Part model, mm, in its own coordinate system. A direction names the side the tool comes from. Give positions to 0.01 mm unless a question says otherwise; leave off trailing zeros. Order: outer loops, then holes, each group sorted by start corner. A loop starts at its lowest first (then second) coordinate and runs counter-clockwise, first axis right, second up. Notation, with made-up numbers: M -24.75,79 L -18.75,79 A12 ccw -18.75,91 Z; hole C 9,75 d7. An arc over 180 degrees is marked long. Return JSON: item names as keys, results as strings.
Autodesk Inventor part; units mm, degrees
ref_plane "YZ Plane" through (0, 0, 0) normal (1, 0, 0) x (0, 1, 0)
ref_plane "XZ Plane" through (0, 0, 0) normal (0, 1, 0) x (-1, 0, 0)
ref_plane "XY Plane" through (0, 0, 0) normal (0, 0, 1) x (1, 0, 0)
sketch "Boceto1" plane through (0, 0, 0) normal (1, 0, 0) x (0, 1, 0)
  line L0 (-6.321, 6.321) -> (6.321, 6.321) construction
  line L1 (6.321, 6.321) -> (6.321, -6.321) construction
  line L2 (6.321, -6.321) -> (-6.321, -6.321) construction
  line L3 (-6.321, -6.321) -> (-6.321, 6.321) construction
  line L4 (-6.321, 6.321) -> (6.321, -6.321) construction
  line L5 (6.321, 6.321) -> (-6.321, -6.321) construction
  circle A0 centre (6.321, -6.321) radius 0.875
  line L6 (0, 0) -> (7.9878, 0) construction
  circle A1 centre (6.321, 6.321) radius 0.875
  line L7 (0, 0) -> (0, -13.4562) construction
  circle A2 centre (-6.321, -6.321) radius 0.875
  circle A3 centre (-6.321, 6.321) radius 0.875
  circle A4 centre (0, 0) radius 5.5
  line L8 (10, 20) -> (-20, 20)
  line L9 (-20, 20) -> (-20, -20)
  line L10 (-20, -20) -> (10, -20)
  line L11 (10, -20) -> (10, 20)
  dimension "d0" = 12.642
  dimension "d1" = 12.642
  dimension "d2" = 1.75
  dimension "d3" = 11
  dimension "d4" = 30
  dimension "d6" = 20
  dimension "d7" = 10
  dimension "d26" = 20
extrude "Extrusión1" add sketch "Boceto1" along normal blind 2
sketch "Boceto2" plane through (0, -20, -20) normal (0, -1, 0) x (1, 0, 0)
  line L0 (2, 0) -> (2, 40)
  line L1 (2, 40) -> (-28, 40)
  line L2 (-28, 40) -> (-28, 0)
  line L3 (-28, 0) -> (2, 0)
  line L4 (2, 0) -> (2, 40)
  point P0 (0, 20)
  point P1 (2, 0)
  dimension "d10" = 30
  dimension "d11" = 40
extrude "Extrusión2" add sketch "Boceto2" along normal blind 2
sketch "Boceto3" plane through (0, -20, -20) normal (0, 1, 0) x (1, 0, 0)
  line L0 (0, -40) -> (0, 0)
  line L1 (-28, 0) -> (0, 0)
  line L2 (-28, -40) -> (-28, 0)
  line L3 (0, -40) -> (-28, -40)
  line L4 (-6.125, -3.125) -> (-6.125, -36.875) construction
  line L5 (-7.25, -3.125) -> (-7.25, -36.875)
  line L6 (-5, -36.875) -> (-5, -3.125)
  arc A0 (-5, -3.125) -> (-7.25, -3.125) centre (-6.125, -3.125) ccw
  arc A1 (-7.25, -36.875) -> (-5, -36.875) centre (-6.125, -36.875) ccw
  line L7 (-21.875, -3.125) -> (-21.875, -36.875) construction
  line L8 (-23, -3.125) -> (-23, -36.875)
  line L9 (-20.75, -36.875) -> (-20.75, -3.125)
  arc A2 (-20.75, -3.125) -> (-23, -3.125) centre (-21.875, -3.125) ccw
  arc A3 (-23, -36.875) -> (-20.75, -36.875) centre (-21.875, -36.875) ccw
  point P0 (0, -20)
  point P1 (-6.125, -20)
  point P2 (-21.875, -20)
  point P3 (-21.875, -38)
  point P4 (-21.875, -2)
  point P5 (-6.125, -38)
  point P6 (-6.125, -2)
  dimension "d14" = 2.25
  dimension "d15" = 2.25
  dimension "d16" = 5
  dimension "d17" = 2
  dimension "d18" = 2
  dimension "d19" = 2
  dimension "d20" = 2
  dimension "d21" = 5
extrude "Extrusión3" cut sketch "Boceto3" against normal through all contours A0 L6 A1 L5 | A2 L9 A3 L8
fillet "Empalme1" radius 1.5 1 edges at (0, -20, 0)
fillet "Empalme2" radius 1 5 edges at (1, 10, 20) (1, 10, -20) (-28, -21, 20) (-28, -21, -20) (2, -22, 0)
properties part number "BRACKET__MOTOR"
Q1. Two-plate mould, pull along Z, no slides. Class faces 1 (the cylindrical face through (-0.43, -19.55, -0.28)), 2 (the flat face through (-5, -21, 0)), 3 (the cylindrical face through (-27.699, -21.014, 19.715)): +Z half, -Z half, draft (parallel to the pull), parting line (faces both ways), or undercut.
Established:
{"face 1": "draft", "face 2": "undercut", "face 3": "+Z half"}
Q2. Pin check, flat tips, straight feed: pin 1 (1.5 mm diameter, centred on y = -16.5, z = 3, fed in from -X); pin 2 (13 mm diameter, centred on x = -12, z = -0.5, fed in from +Y). Stop position of each tip, or through.
Established:
{"pin 1": "stops at x = 0", "pin 2": "stops at y = -20"}
Q3. Band-saw the part on D-D (x = -21.75). Give the cut face in (y, z), then the cut area to 3 significant figures.
Established:
{"outline": "M -22,-20 L -20,-20 L -20,-17.99 L -22,-17.99 Z; M -22,17.99 L -20,17.99 L -20,20 L -22,20 Z", "area": "8.03 mm²"}
Q4. Band-saw the part on A-A (y = 0). Give the cut face in (x, z), then the cut area to 3 significant figures.
Established:
{"outline": "M 0,-20 L 2,-20 L 2,-5.5 L 0,-5.5 Z; M 0,5.5 L 2,5.5 L 2,20 L 0,20 Z", "area": "58.0 mm²"}
Q5. 3-axis set-ups, long thin cutter, end or side, ignore diameter. For faces 4 (the cylindrical face through (1.014, 9.715, 19.699)), 5 (the flat face through (-23, -21, 0)): which of +Z, -Z, +X, -X, +Y, -Y reach the whole face in a straight line?
Established:
{"face 4": "+Z, +X, -X, +Y", "face 5": "+Y, -Y"}
Q6. Probe line 1 along Z through (x, y) = (1.4, 0); line 2 along Y through (x, z) = (-1.5, 2); line 3 along X through (y, z) = (-16, 17.5). List the from-to ranges inside material, lowest first.
Established:
{"line 1": "z = -20 to -5.5, 5.5 to 20", "line 2": "y = -22 to -20", "line 3": "x = 0 to 2"}
Q7. Band-saw the part on C-C (z = 8.5). Give the cut face in (x, y).
Established:
{"outline": "M -28,-22 L -23,-22 L -23,-20 L -28,-20 Z; M -20.75,-22 L -7.25,-22 L -7.25,-20 L -20.75,-20 Z; M -5,-22 L 1,-22 A1 ccw 2,-21 L 2,10 L 0,10 L 0,-18.5 A1.5 cw -1.5,-20 L -5,-20 Z"}
Q8. Band-saw the part on B-B (z = 0). Give the cut face in (x, y), then the cut area to 3 significant figures.
Established:
{"outline": "M -28,-22 L -23,-22 L -23,-20 L -28,-20 Z; M -20.75,-22 L -7.25,-22 L -7.25,-20 L -20.75,-20 Z; M -5,-22 L 1,-22 A1 ccw 2,-21 L 2,-5.5 L 0,-5.5 L 0,-18.5 A1.5 cw -1.5,-20 L -5,-20 Z; M 0,5.5 L 2,5.5 L 2,10 L 0,10 Z", "area": "89.3 mm²"}
